Can you work these out from the drawing? Everything is in mm from the part's minimum corner. Coordinates: 2 decimals unless noted, no trailing zeros. Loops run counter-clockwise (first coordinate to the right, second up) from the corner with the lowest first, then second, coordinate; pieces in that order, holes last. Notation, with made-up numbers: (11, -23.75) -> (39, -23.75) arc R19 cw to (39, 8.25) -> close; hole circle Ø7 at (31.5, 3). An arc over 180 degrees is marked (long way). One line per question, with ' | ' between items.
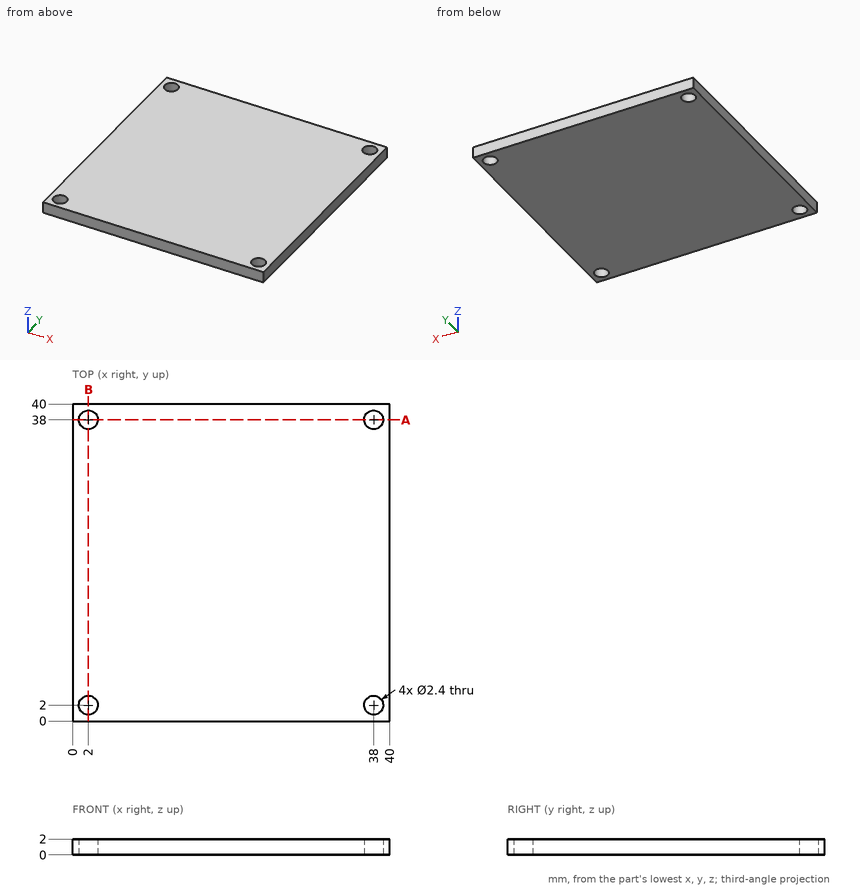
Q1. Imagine slicing it at A-A on y = 38. Write out the boundary of the cut face in (x, z).
Values follow:
outline: (0, 0) -> (0.8, 0) -> (0.8, 2) -> (0, 2) -> close; (3.2, 0) -> (36.8, 0) -> (36.8, 2) -> (3.2, 2) -> close; (39.2, 0) -> (40, 0) -> (40, 2) -> (39.2, 2) -> close
Q2. Please list where this line runs through material, in increasing order: L1, parallel to Y at x = 2, z = 0.5. Write a range as [from, to].
Values follow:
L1: y = [0, 0.8], [3.2, 36.8], [39.2, 40]
Q3. For pin 1 (1 mm diameter, centred on x = 9, y = 24.5, fed in from -Z), with a flat end and sliding along its axis, tell me the tip position at first contact or that it passes through.
Values follow:
pin 1: stops at z = 0
